Model file for the job. Use its own axes, mm. A direction names the side the tool comes from. Round coordinates to 2 decimals unless told otherwise and drop trailing zeros. Order: outer loops, then holes, each group sorted by start corner. A loop starts at its lowest first (then second) coordinate and runs counter-clockwise, first axis right, second up. Notation, with made-up numbers: (-24.5, 75.5) -> (-3.5, 75.5) arc R34 ccw to (-3.5, 113.5) -> close; hole circle Ø8 at (48.5, -26.75). An arc over 180 degrees is marked (long way). Put each result on its own line as item: value. Start each with the question number.
Q1. Pull direction X, two halves, no side cores. Call faces 1 (the face through (3.543, 5.708, 1.109)), 2 (the face through (-20, 0, 1)), 3 (the face through (-13.98, 8.15, 3.18)): released by +X, released by -X, zero draft, split by the parting line, or undercut.
Q2. 3-axis set-ups, long thin cutter, end or side, ignore diameter. For faces 4 (the face through (6.75, 3, 1)), 5 (the face through (19, -4.25, 1)), 6 (the face through (-9.25, -4, 1)): which of +Z, -Z, +X, -X, +Y, -Y reach the whole face in a straight line?
Q3. Cut at A-A, the plane y = -0.25. List the corners of the cut face in (x, z), and give its area (3 significant figures).
Q4. Flat gauge pins, fed straight in: P1, Ø1.5, axis at x = -15.5, z = 3, coming from the +Y side; P2, Ø2, axis at x = 1.5, y = -6, coming from the +Z side; P3, Ø1.1, axis at x = 19, z = 1, coming from the +Y side. Where does each tip first touch, or does it go through?
Q5. Cut at C-C, the plane x = -5.5. List the corners of the cut face in (y, z).
Q6. Probe L1, parallel to X at y = -8, z = 1.85; L2, parallel to X at y = -6, z = 0.45; L3, parallel to X at y = 6.25, z = 1.55. List the from-to ranges inside material, lowest first.
Q7. Cut at B-B, the plane z = 3.1. List the corners of the cut face in (x, y).
from build123d import *
from OCP.BRepFilletAPI import BRepFilletAPI_MakeChamfer

# Parameters (mm, degrees)
ESBO_O10_W               = 40
ESBO_O10_H               = 17.5
RESSALTO_EXTRUS_O6_DEPTH = 2.25
CORTE_EXTRUS_O2_DEPTH    = 2.5
ESBO_O12_W               = 3.5
ESBO_O12_H               = 2.75
RESSALTO_EXTRUS_O7_DEPTH = 1.5
ESBO_O13_W               = 3
ESBO_O13_H               = 1.5
ESBO_O13_W_2             = 2
CORTE_EXTRUS_O3_DEPTH    = 8
CORTE_EXTRUS_O4_DEPTH    = 20
CHANFRO5_SIZE            = 6
CHANFRO5_SIZE_2          = 0.419560872
CHANFRO6_SIZE            = 1
CHANFRO6_SIZE2           = 0.839099631
FILETE1_R                = 2


with BuildPart() as part:
    # Esboço10 → Ressalto-extrusão6 (new body)
    with BuildSketch(Plane.XY):
        Rectangle(ESBO_O10_W, ESBO_O10_H)
    extrude(amount=RESSALTO_EXTRUS_O6_DEPTH)

    # Esboço11 → Corte-extrusão2 (cut)
    with BuildSketch(Plane.XY.offset(2.25)):
        Polygon((-20, 3.75), (-15.75, 3.75), (-15.75, 8.75), (-12.25, 8.75), (-12.25, 3.75), (-3.75, 3.75), (-3.75, 9.75), (3.75, 9.75), (3.75, 3.75), (12.25, 3.75), (12.25, 8.75), (15.75, 8.75), (15.75, 3.75), (20, 3.75), (20, 11.902365005), (-20, 11.902365005), align=None)
        Polygon((-20, -4.25), (-15.75, -4.25), (-15.75, -8.75), (-12.25, -8.75), (-12.25, -4.25), (-3.75, -4.25), (-3.75, -10.25), (3.75, -9.74672567), (3.75, -4.25), (12.25, -4.25), (12.25, -8.75), (15.75, -8.75), (15.75, -4.25), (20, -4.25), (20, -11.31917021), (-20, -11.31917021), align=None)
    extrude(amount=-CORTE_EXTRUS_O2_DEPTH, mode=Mode.SUBTRACT)

    # Esboço12 → Ressalto-extrusão7 (add)
    with BuildSketch(Plane.XY.offset(2.25)):
        with Locations((-14, 7.375)):
            Rectangle(ESBO_O12_W, ESBO_O12_H)
        with Locations((-14, -7.375)):
            Rectangle(ESBO_O12_W, ESBO_O12_H)
        with Locations((14, -7.375)):
            Rectangle(ESBO_O12_W, ESBO_O12_H)
        with Locations((14, 7.375)):
            Rectangle(ESBO_O12_W, ESBO_O12_H)
    extrude(amount=RESSALTO_EXTRUS_O7_DEPTH)

    # Esboço13 → Corte-extrusão3 (cut)
    with BuildSketch(Plane.XY.offset(2.25)):
        with Locations((-10.75, 3)):
            Rectangle(ESBO_O13_W, ESBO_O13_H)
        with Locations((-5.25, 3)):
            Rectangle(ESBO_O13_W, ESBO_O13_H)
        with Locations((5.25, 3)):
            Rectangle(ESBO_O13_W, ESBO_O13_H)
        with Locations((10.75, 3)):
            Rectangle(ESBO_O13_W, ESBO_O13_H)
        with Locations((10.75, -3.5)):
            Rectangle(ESBO_O13_W, ESBO_O13_H)
        with Locations((5.25, -3.5)):
            Rectangle(ESBO_O13_W, ESBO_O13_H)
        with Locations((-5.25, -3.5)):
            Rectangle(ESBO_O13_W, ESBO_O13_H)
        with Locations((-10.75, -3.5)):
            Rectangle(ESBO_O13_W, ESBO_O13_H)
        with Locations((-16.75, -3.5)):
            Rectangle(ESBO_O13_W_2, ESBO_O13_H)
        with Locations((-16.75, 3)):
            Rectangle(ESBO_O13_W_2, ESBO_O13_H)
        with Locations((16.75, 3)):
            Rectangle(ESBO_O13_W_2, ESBO_O13_H)
        with Locations((16.75, -3.5)):
            Rectangle(ESBO_O13_W_2, ESBO_O13_H)
    extrude(amount=-CORTE_EXTRUS_O3_DEPTH, mode=Mode.SUBTRACT)

    # Esboço15 → Corte-extrusão4 (cut)
    with BuildSketch(Plane.XY.offset(2.25)):
        Polygon((-1.75, 5.75), (1.75, 5.75), (1.75, -5.75), (0, -7.015048633), (-1.75, -5.75), align=None)
    extrude(amount=-CORTE_EXTRUS_O4_DEPTH, mode=Mode.SUBTRACT)

    # Chanfro5
    chanfro5_edges_1 = [part.edges().sort_by_distance(p)[0] for p in [
        (-15.75, -8.75, 1.875),
    ]]
    chanfro5_side_1 = [part.faces().sort_by_distance(p)[0] for p in [
        (-15.75, -8.741608783, 1.875),
    ]]
    chanfro5_edges_2 = [part.edges().sort_by_distance(p)[0] for p in [
        (-3.75, -8.75, 1.125),
    ]]
    chanfro5_side_2 = [part.faces().sort_by_distance(p)[0] for p in [
        (-3.75, -8.741608783, 1.125),
    ]]
    chanfro5_edges_3 = [part.edges().sort_by_distance(p)[0] for p in [
        (12.25, -8.75, 1.875),
    ]]
    chanfro5_side_3 = [part.faces().sort_by_distance(p)[0] for p in [
        (12.25, -8.741608783, 1.875),
    ]]
    chanfro5_edges_4 = [part.edges().sort_by_distance(p)[0] for p in [
        (15.75, 8.75, 1.875),
    ]]
    chanfro5_side_4 = [part.faces().sort_by_distance(p)[0] for p in [
        (15.741608783, 8.75, 1.875),
    ]]
    chanfro5_edges_5 = [part.edges().sort_by_distance(p)[0] for p in [
        (3.75, 8.75, 1.125),
    ]]
    chanfro5_side_5 = [part.faces().sort_by_distance(p)[0] for p in [
        (3.741608783, 8.75, 1.125),
    ]]
    chanfro5_edges_6 = [part.edges().sort_by_distance(p)[0] for p in [
        (-12.25, 8.75, 1.875),
    ]]
    chanfro5_side_6 = [part.faces().sort_by_distance(p)[0] for p in [
        (-12.258391217, 8.75, 1.875),
    ]]
    chanfro5_edges_7 = [part.edges().sort_by_distance(p)[0] for p in [
        (-12.25, -8.75, 1.875),
    ]]
    chanfro5_side_7 = [part.faces().sort_by_distance(p)[0] for p in [
        (-12.258391217, -8.75, 1.875),
    ]]
    chanfro5_edges_8 = [part.edges().sort_by_distance(p)[0] for p in [
        (3.75, -8.75, 1.125),
    ]]
    chanfro5_side_8 = [part.faces().sort_by_distance(p)[0] for p in [
        (3.741608783, -8.75, 1.125),
    ]]
    chanfro5_edges_9 = [part.edges().sort_by_distance(p)[0] for p in [
        (15.75, -8.75, 1.875),
    ]]
    chanfro5_side_9 = [part.faces().sort_by_distance(p)[0] for p in [
        (15.741608783, -8.75, 1.875),
    ]]
    chanfro5_edges_10 = [part.edges().sort_by_distance(p)[0] for p in [
        (12.25, 8.75, 1.875),
    ]]
    chanfro5_side_10 = [part.faces().sort_by_distance(p)[0] for p in [
        (12.25, 8.741608783, 1.875),
    ]]
    chanfro5_edges_11 = [part.edges().sort_by_distance(p)[0] for p in [
        (-3.75, 8.75, 1.125),
    ]]
    chanfro5_side_11 = [part.faces().sort_by_distance(p)[0] for p in [
        (-3.75, 8.741608783, 1.125),
    ]]
    chanfro5_edges_12 = [part.edges().sort_by_distance(p)[0] for p in [
        (-15.75, 8.75, 1.875),
    ]]
    chanfro5_side_12 = [part.faces().sort_by_distance(p)[0] for p in [
        (-15.741608783, 8.75, 1.875),
    ]]
    chanfro5 = BRepFilletAPI_MakeChamfer(part.part.solid().wrapped)
    for e in chanfro5_edges_1:
        chanfro5.Add(CHANFRO5_SIZE - 0.0001, CHANFRO5_SIZE_2 - 0.0001, e.wrapped, chanfro5_side_1[0].wrapped)
    for e in chanfro5_edges_2:
        chanfro5.Add(CHANFRO5_SIZE - 0.0001, CHANFRO5_SIZE_2 - 0.0001, e.wrapped, chanfro5_side_2[0].wrapped)
    for e in chanfro5_edges_3:
        chanfro5.Add(CHANFRO5_SIZE - 0.0001, CHANFRO5_SIZE_2 - 0.0001, e.wrapped, chanfro5_side_3[0].wrapped)
    for e in chanfro5_edges_4:
        chanfro5.Add(CHANFRO5_SIZE_2 - 0.0001, CHANFRO5_SIZE - 0.0001, e.wrapped, chanfro5_side_4[0].wrapped)
    for e in chanfro5_edges_5:
        chanfro5.Add(CHANFRO5_SIZE_2 - 0.0001, CHANFRO5_SIZE - 0.0001, e.wrapped, chanfro5_side_5[0].wrapped)
    for e in chanfro5_edges_6:
        chanfro5.Add(CHANFRO5_SIZE_2 - 0.0001, CHANFRO5_SIZE - 0.0001, e.wrapped, chanfro5_side_6[0].wrapped)
    for e in chanfro5_edges_7:
        chanfro5.Add(CHANFRO5_SIZE_2 - 0.0001, CHANFRO5_SIZE - 0.0001, e.wrapped, chanfro5_side_7[0].wrapped)
    for e in chanfro5_edges_8:
        chanfro5.Add(CHANFRO5_SIZE_2 - 0.0001, CHANFRO5_SIZE - 0.0001, e.wrapped, chanfro5_side_8[0].wrapped)
    for e in chanfro5_edges_9:
        chanfro5.Add(CHANFRO5_SIZE_2 - 0.0001, CHANFRO5_SIZE - 0.0001, e.wrapped, chanfro5_side_9[0].wrapped)
    for e in chanfro5_edges_10:
        chanfro5.Add(CHANFRO5_SIZE - 0.0001, CHANFRO5_SIZE_2 - 0.0001, e.wrapped, chanfro5_side_10[0].wrapped)
    for e in chanfro5_edges_11:
        chanfro5.Add(CHANFRO5_SIZE - 0.0001, CHANFRO5_SIZE_2 - 0.0001, e.wrapped, chanfro5_side_11[0].wrapped)
    for e in chanfro5_edges_12:
        chanfro5.Add(CHANFRO5_SIZE_2 - 0.0001, CHANFRO5_SIZE - 0.0001, e.wrapped, chanfro5_side_12[0].wrapped)
    add(Compound.cast(chanfro5.Shape()), mode=Mode.REPLACE)  # a hair under: the kernel refuses the full size

    # Chanfro6: one chamfer whose edges measure the first distance from different faces: ONE call of the kernel's chamfer builder (chamfer() names one face for all edges)
    chanfro6_edges_1 = [part.edges().sort_by_distance(p)[0] for p in [
        (0, -8.75, 2.25),
    ]]
    chanfro6_side_1 = [part.faces().sort_by_distance(p)[0] for p in [
        (0, -8.75, 1.125),
    ]]
    chanfro6_edges_2 = [part.edges().sort_by_distance(p)[0] for p in [
        (0, 8.75, 2.25),
    ]]
    chanfro6_side_2 = [part.faces().sort_by_distance(p)[0] for p in [
        (0, 8.75, 1.125),
    ]]
    chanfro6 = BRepFilletAPI_MakeChamfer(part.part.solid().wrapped)
    for e in chanfro6_edges_1:
        chanfro6.Add(CHANFRO6_SIZE, CHANFRO6_SIZE2, e.wrapped, chanfro6_side_1[0].wrapped)  # the first distance lies on this face
    for e in chanfro6_edges_2:
        chanfro6.Add(CHANFRO6_SIZE, CHANFRO6_SIZE2, e.wrapped, chanfro6_side_2[0].wrapped)  # the first distance lies on this face
    add(Compound.cast(chanfro6.Shape()), mode=Mode.REPLACE)

    # Filete1
    filete1_edges = [part.edges().sort_by_distance(p)[0] for p in [
        (-14, -8.75, 3.75),
        (14, -8.75, 3.75),
        (14, 8.75, 3.75),
        (-14, 8.75, 3.75),
    ]]
    fillet(filete1_edges, radius=FILETE1_R)


solid = part.part
Ans:
1. face 1: undercut
1. face 2: released by -X
1. face 3: zero draft
2. face 4: +Z, -Z, +Y
2. face 5: +Z, -Z, +X, -Y
2. face 6: +Z, -Z, -Y
3. outline: (-20, 0) -> (-1.75, 0) -> (-1.75, 2.25) -> (-20, 2.25) -> close; (1.75, 0) -> (20, 0) -> (20, 2.25) -> (1.75, 2.25) -> close
3. area: 82.1 mm^2
4. P1: stops at y = 8.68
4. P2: stops at z = 2.25
4. P3: stops at y = 3.75
5. outline: (-2.75, 0) -> (2.25, 0) -> (2.25, 2.25) -> (-2.75, 2.25) -> close
6. L1: x = -15.38 to -12.62, -3.38 to 3.38, 12.62 to 15.38
6. L2: x = -15.52 to -12.48, -3.52 to -1.4, 1.4 to 3.52, 12.48 to 15.52
6. L3: x = -15.51 to -12.49, -3.51 to 3.51, 12.49 to 15.51
7. outline: (-15.52, -6) -> (-15.37, -8.23) -> (-12.63, -8.23) -> (-12.48, -6) -> close; (-15.52, 6) -> (-12.48, 6) -> (-12.63, 8.23) -> (-15.37, 8.23) -> close; (12.48, -6) -> (12.63, -8.23) -> (15.37, -8.23) -> (15.52, -6) -> close; (12.48, 6) -> (15.52, 6) -> (15.37, 8.23) -> (12.63, 8.23) -> close
